Read the model definition and answer for the solid it produces. Units are mm, in the model's axes. A direction names the side the tool comes from. Coordinates: 2 decimals unless noted, no trailing zeros. Write each loop counter-clockwise with the first axis right and the second up, starting at its lowest first coordinate (ties: lowest second). Pieces come first, ordered by that corner, then holes. Notation, with made-up numbers: (26.5, 15.5) -> (48.5, 15.5) arc R27 cw to (48.5, 48.5) -> close; hole circle Ø10 at (14.5, 9). An arc over 180 degrees is marked (long way). Use CSV: the item, a comma, the result in double quotes.
Autodesk Fusion 360 part; units mm, degrees
sketch "Sketch1" plane through (0, 0, 0) normal (0, 0, 1) x (1, 0, 0)
  line L0 (0, 0) -> (-65, 0)
  line L1 (-65, 0) -> (-65, -5)
  line L2 (-65, -5) -> (-73, 1.6)
  line L3 (-73, 1.6) -> (-2, 4)
  line L4 (-2, 4) -> (-2, 15)
  line L5 (-2, 15) -> (0, 15)
  line L6 (0, 15) -> (0, 0)
  line L7 (-2, 4) -> (-2, 0)
  dimension "d1" = 65
  dimension "d2" = 15
  dimension "d3" = 2
  dimension "d4" = 5
  dimension "d5" = 8
  dimension "d6" = 1.6
  dimension "d7" = 4
extrude "Extrude1" add sketch "Sketch1" along normal blind 15 contours L0 L4 L5 L6 L7
extrude "Extrude2" add sketch "Sketch1" along normal blind 10 contours L0 L1 L2 L3 L7
sketch "Sketch2" plane through (0, 0, 0) normal (1, 0, 0) x (0, 1, 0)
  line L0 (0, 0) -> (15, 0)
  line L1 (15, 0) -> (15, 15)
  line L2 (15, 15) -> (0, 15)
  line L3 (0, 15) -> (0, 0)
  line L4 (4, 10) -> (0, 10) construction
  line L5 (4, 0) -> (4, 10) construction
  line L6 (3.75, 10.5322) -> (11.25, 10.5322)
  arc A0 (11.25, 10.5322) -> (11.25, 14.0322) centre (11.25, 12.2822) ccw
  line L7 (11.25, 14.0322) -> (3.75, 14.0322)
  arc A1 (3.75, 14.0322) -> (3.75, 10.5322) centre (3.75, 12.2822) ccw
  line L8 (3.75, 12.2822) -> (11.25, 12.2822) construction
  line L9 (7.5, 15) -> (7.5, 0) construction
  line L10 (7.75, 2.9241) -> (11.25, 2.9241)
  arc A2 (11.25, 2.9241) -> (11.25, 6.4241) centre (11.25, 4.6741) ccw
  line L11 (11.25, 6.4241) -> (7.75, 6.4241)
  arc A3 (7.75, 6.4241) -> (7.75, 2.9241) centre (7.75, 4.6741) ccw
  line L12 (6, 4.6741) -> (13, 4.6741) construction
  dimension "d12" = 3.5
  dimension "d13" = 3.5
  dimension "d14" = 2
  dimension "d15" = 2
  dimension "d16" = 2
  dimension "d17" = 2
extrude "Extrude3" cut sketch "Sketch2" against normal up to surface (2 mm away) contours L6 A0 L7 A1 | L10 A2 L11 A3
fillet "Fillet1" radius 1 1 edges at (-2, 4, 5)
equation "d13 = d12"
1. A cutting plane is placed at B-B (z = 4). Give the vertices of the cut face in (x, y).
Solutions:
outline,"(-73, 1.6) -> (-65, -5) -> (-65, 0) -> (0, 0) -> (0, 6.14) -> (-2, 6.14) -> (-2, 4.97) arc R1 cw to (-2.97, 3.97) -> close; (-2, 12.86) -> (0, 12.86) -> (0, 15) -> (-2, 15) -> close"
2. Each of these flat-tipped pins is pushed along its axis until it touches: pin 1 Ø3 at (x, y) = (-22, 0.5) entering from +Z; pin 2 Ø8 at (y, z) = (3.5, 9) entering from +X; pin 3 Ø2 at (y, z) = (5.5, 6) entering from -X; pin 4 Ø3 at (x, z) = (-31, 8) entering from +Y. Where does it stop, or does it pass through?
Solutions:
pin 1,"stops at z = 10"
pin 2,"stops at x = 0"
pin 3,"stops at x = -2.12"
pin 4,"stops at y = 3.07"
3. A cutting plane is placed at C-C (z = 7.75). Give the vertices of the cut face in (x, y).
Solutions:
outline,"(-73, 1.6) -> (-65, -5) -> (-65, 0) -> (0, 0) -> (0, 15) -> (-2, 15) -> (-2, 4.97) arc R1 cw to (-2.97, 3.97) -> close"
4. For a pull along Y with two mould halves and no side action, classify faces 5 (the flat face through (-1, 8, 14.032)), 6 (the flat face through (-65, -2, 5)), 7 (the cylindrical face through (-1, 2, 12.3)), 8 (the flat face through (-1, 15, 7)) as pulls with the +Y half, pulls with the -Y half, needs draft (parallel to the pull), parting line crosses it, or undercut.
Solutions:
face 5,"undercut"
face 6,"needs draft"
face 7,"undercut"
face 8,"pulls with the +Y half"
5. A cutting plane is placed at A-A (y = 9.5). Give the vertices of the cut face in (x, z), and give its area (3 significant figures).
Solutions:
outline,"(-2, 0) -> (0, 0) -> (0, 2.92) -> (-2, 2.92) -> close; (-2, 6.42) -> (0, 6.42) -> (0, 10.53) -> (-2, 10.53) -> close; (-2, 14.03) -> (0, 14.03) -> (0, 15) -> (-2, 15) -> close"
area,"16.0 mm^2"
6. A cutting plane is placed at D-D (x = -61). Give the vertices of the cut face in (y, z).
Solutions:
outline,"(0, 0) -> (2.01, 0) -> (2.01, 10) -> (0, 10) -> close"
7. Find the intervals of material crossed by line 1 along X through (y, z) = (1, 13.5); line 2 along Z through (x, y) = (-34, 0.75); line 3 along Y through (x, z) = (-42, 5.25), in increasing order.
Solutions:
line 1,"x = -2 to 0"
line 2,"z = 0 to 10"
line 3,"y = 0 to 2.65"
8. A tool of negligible diameter and unlimited length cuts with its end or side. For faces 1 (the flat face through (-2, 9, 7)), 2 (the flat face through (-35, 1, 10)), 3 (the flat face through (-32, 0, 4)), 4 (the cylindrical face through (-1, 13, 4.6)), from which of +Z, -Z, +X, -X, +Y, -Y can it reach the whole face along a straight path? Write none if from no direction.
Solutions:
face 1,"+Z, -X, +Y"
face 2,"+Z, -X, +Y, -Y"
face 3,"+Z, -Z, +X, -Y"
face 4,"+X, -X"
